Check sheet for the modelled part. Datum: model origin and axes. Units: mm. Face numbers are marked on the shaded views. A direction names the side the tool comes from. Round coordinates to 2 decimals unless told otherwise and drop trailing zeros. Write each loop counter-clockwise with the first axis right and the second up, starting at its lowest first coordinate (ties: lowest second). Pieces come first, ordered by that corner, then holes. Notation, with made-up numbers: (-32.75, 64) -> (-22.75, 64) arc R20 cw to (-22.75, 78) -> close; hole circle Ø10 at (-18.75, 80). An arc over 180 degrees is marked (long way). Write item = value, one per line.
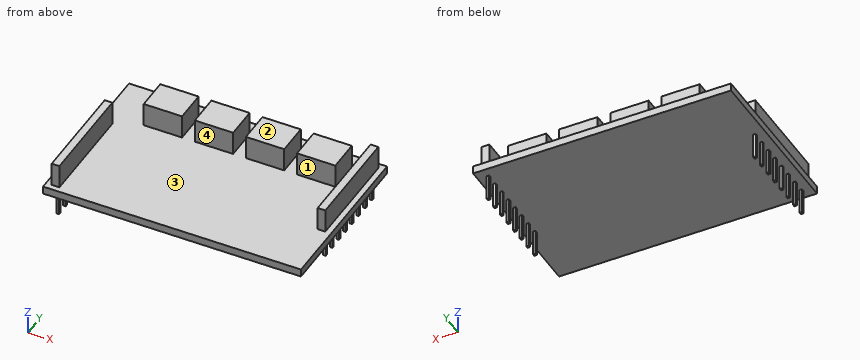
from build123d import *

# Parameters (mm, degrees)
SKETCH1_W           = 51.308
SKETCH1_H           = 33.02
BOSS_EXTRUDE1_DEPTH = 1.5748
SKETCH2_W           = 1.524
SKETCH2_H           = 20.32
BOSS_EXTRUDE2_DEPTH = 6.35
SKETCH3_W           = 7.62
SKETCH3_H           = 6.35
BOSS_EXTRUDE3_DEPTH = 6.35
LPATTERN2_COUNT     = 4
LPATTERN2_PITCH     = 10.16
SKETCH6_W           = 0.508
SKETCH6_H           = 0.508
BOSS_EXTRUDE4_DEPTH = 5.08
LPATTERN3_COUNT     = 8
LPATTERN3_PITCH     = 2.54
SKETCH7_W           = 0.508
SKETCH7_H           = 0.508
BOSS_EXTRUDE5_DEPTH = 5.08
LPATTERN4_COUNT     = 8
LPATTERN4_PITCH     = 2.54


with BuildPart() as part:
    # Sketch1 → Boss-Extrude1 (new body)
    with BuildSketch(Plane.XY):
        with Locations((25.654, 16.51)):
            Rectangle(SKETCH1_W, SKETCH1_H)
    extrude(amount=BOSS_EXTRUDE1_DEPTH)

    # Sketch2 → Boss-Extrude2 (add)
    with BuildSketch(Plane.XY):
        with Locations((49.403, 21.717)):
            Rectangle(SKETCH2_W, SKETCH2_H)
        with Locations((1.905, 11.303)):
            Rectangle(SKETCH2_W, SKETCH2_H)
    extrude(amount=BOSS_EXTRUDE2_DEPTH)

    # Sketch3 → Boss-Extrude3 (add)
    with BuildSketch(Plane.XY):
        with Locations((11.577275474, 26.851190856)):
            Rectangle(SKETCH3_W, SKETCH3_H)
    boss_extrude3 = extrude(amount=BOSS_EXTRUDE3_DEPTH)

    # LPattern2: Boss-Extrude3 ×4
    with Locations(*[(i * LPATTERN2_PITCH, 0, 0) for i in range(1, LPATTERN2_COUNT)]):
        add(boss_extrude3)

    # Sketch6 → Boss-Extrude4 (add)
    with BuildSketch(Plane(origin=(0, 0, 0), x_dir=(-1, 0, 0), z_dir=(0, 0, -1))):
        with Locations((-49.276, 30.978319105)):
            Rectangle(SKETCH6_W, SKETCH6_H)
    boss_extrude4 = extrude(amount=BOSS_EXTRUDE4_DEPTH)

    # LPattern3: Boss-Extrude4 ×8
    with Locations(*[(0, -i * LPATTERN3_PITCH, 0) for i in range(1, LPATTERN3_COUNT)]):
        add(boss_extrude4)

    # Sketch7 → Boss-Extrude5 (add)
    with BuildSketch(Plane(origin=(0, 0, 0), x_dir=(-1, 0, 0), z_dir=(0, 0, -1))):
        with Locations((-2.032, 2.032)):
            Rectangle(SKETCH7_W, SKETCH7_H)
    boss_extrude5 = extrude(amount=BOSS_EXTRUDE5_DEPTH)

    # LPattern4: Boss-Extrude5 ×8
    with Locations(*[(0, i * LPATTERN4_PITCH, 0) for i in range(1, LPATTERN4_COUNT)]):
        add(boss_extrude5)


solid = part.part
(1) Sectioned sample at A-A on z = 4.75. Enter the section's corners in (x, y) (3 decimals), then the cut area to 3 significant figures.
Worked answers:
outline = (1.143, 1.143) -> (2.667, 1.143) -> (2.667, 21.463) -> (1.143, 21.463) -> close; (7.767, 23.676) -> (15.387, 23.676) -> (15.387, 30.026) -> (7.767, 30.026) -> close; (17.927, 23.676) -> (25.547, 23.676) -> (25.547, 30.026) -> (17.927, 30.026) -> close; (28.087, 23.676) -> (35.707, 23.676) -> (35.707, 30.026) -> (28.087, 30.026) -> close; (38.247, 23.676) -> (45.867, 23.676) -> (45.867, 30.026) -> (38.247, 30.026) -> close; (48.641, 11.557) -> (50.165, 11.557) -> (50.165, 31.877) -> (48.641, 31.877) -> close
area = 255 mm²
(2) Sectioned sample at B-B on y = 3.5. Enter the section's corners in (x, z), then the cut area to 3 significant figures.
Worked answers:
outline = (0, 0) -> (51.31, 0) -> (51.31, 1.57) -> (2.67, 1.57) -> (2.67, 6.35) -> (1.14, 6.35) -> (1.14, 1.57) -> (0, 1.57) -> close
area = 88.1 mm²
(3) Go/stop test with flat-tipped pins: P1, Ø2.5, axis at y = 20.5, z = 3, coming from the +X side (3 decimals); P2, Ø5.5, axis at y = 27, z = 4.5, coming from the -X side; P3, Ø0.6, axis at x = 49.5, z = -1.5, coming from the -Y side. Record where each tip stops, or that it passes through.
Worked answers:
P1 = 50.165
P2 = 7.77
P3 = 12.94
(4) Material ranges on L1, parallel to Y at x = 33, z = 5.25; L2, parallel to Z at x = 25.5, y = 27.5; L3, parallel to X at y = 16.5, z = 5 (3 decimals), recorded low to high. Write a range as [from, to].
Worked answers:
L1 = [23.68, 30.03]
L2 = [0, 6.35]
L3 = [1.143, 2.667], [48.641, 50.165]
(5) Sectioned sample at D-D on x = 33. Enter the section's corners in (y, z), then the cut area to 3 significant figures.
Worked answers:
outline = (0, 0) -> (33.02, 0) -> (33.02, 1.57) -> (30.03, 1.57) -> (30.03, 6.35) -> (23.68, 6.35) -> (23.68, 1.57) -> (0, 1.57) -> close
area = 82.3 mm²
(6) Release check for a two-part mould opening along X. For the marked faces 3 and 4 record: pulls with the +X half, pulls with the -X half, needs draft (parallel to the pull), parting line crosses it, or undercut.
Worked answers:
face_3 = undercut
face_4 = needs draft
(7) Sectioned sample at C-C on z = -2.25. Count the separate pieces of the cut face and the enclosed holes in it, then the cut area to 3 significant figures.
Worked answers:
separate_pieces = 16
enclosed_holes = 0
area = 4.13 mm²
(8) Access from +Z, -Z, +X, -X, +Y, -Y to the whole of each face (thin tool, end or side, straight path). Record for the marked faces 1 and 2.
Worked answers:
face_1 = +Z, -X, -Y
face_2 = +Z, +X, -X, +Y, -Y
